Geometry: final body of the model. Coordinates: model frame, mm. A direction names the side the tool comes from. Coordinates: 2 decimals unless noted, no trailing zeros. Order: outer loops, then holes, each group sorted by start corner. A loop starts at its lowest first (then second) coordinate and runs counter-clockwise, first axis right, second up. Notation, with made-up numbers: (61, 85.5) - (80, 85.5) arc R32 ccw to (80, 113.5) - close; hole circle Ø9 at (-2.5, 69.5). An arc over 180 degrees is marked (long way). Use a Markdown table: item, result. Add a question column.
```python
from build123d import *

# Parameters (mm, degrees)
CROQUIS1_W              = 50
CROQUIS1_H              = 50
CROQUIS1_W_2            = 40
CROQUIS1_H_2            = 40
SALIENTE_EXTRUIR1_DEPTH = 25
CROQUIS2_R              = 8
CORTAR_EXTRUIR1_DEPTH   = 60
CROQUIS3_R              = 8
CORTAR_EXTRUIR2_DEPTH   = 60


with BuildPart() as part:
    # Croquis1 → Saliente-Extruir1 (new body)
    with BuildSketch(Plane.XY):
        Rectangle(CROQUIS1_W, CROQUIS1_H)
        Rectangle(CROQUIS1_W_2, CROQUIS1_H_2, mode=Mode.SUBTRACT)
    extrude(amount=SALIENTE_EXTRUIR1_DEPTH)

    # Croquis2 → Cortar-Extruir1 (cut)
    with BuildSketch(Plane(origin=(0, 25, 0), x_dir=(1, 0, 0), z_dir=(0, 1, 0))):
        with Locations(Location((0, -12.5, 0), (0, 0, 270))):
            Circle(CROQUIS2_R)
    extrude(amount=-CORTAR_EXTRUIR1_DEPTH, mode=Mode.SUBTRACT)

    # Croquis3 → Cortar-Extruir2 (cut)
    with BuildSketch(Plane(origin=(25, 0, 0), x_dir=(0, 0, -1), z_dir=(1, 0, 0))):
        with Locations(Location((-12.5, 0, 0), (0, 0, 90))):
            Circle(CROQUIS3_R)
    extrude(amount=-CORTAR_EXTRUIR2_DEPTH, mode=Mode.SUBTRACT)


solid = part.part
```
1) Section query A-A (x = 0). Return the cut outline in (y, z).
2) Line query: line 1 (Y direction, x = -9, z = 15.5); line 2 (X direction, y = -22.55, z = 12.5). Output: solid intervals per line, ascending. Write a range as from..to.
3) Access query for faces 4 (the cylindrical face through (-22.47, -1.73, 4.69)), 5 (the flat face through (0, -20, 21)). Directions: +Z, -Z, +X, -X, +Y, -Y. A direction counts if a zero-diameter tool reaches every point of the face in a straight line with its end or side. Return the directions, or none.
4) Section query B-B (y = 12). Return the cut outline in (x, z).
5) Draft query along Z for faces 1 (the flat face through (-23, 0, 0)), 2 (the flat face through (-5.9, 25, 6.8)), 3 (the cylindrical face through (-7.81, 22.54, 10.77)). Return one class per face: released by +Z, released by -Z, zero draft, split by the parting line, or undercut.
6) Section query D-D (z = 12.5). Return the cut outline in (x, y).
From the geometry:
| question | item | result |
|---|---|---|
| 1 | outline | (-25, 0) - (-20, 0) - (-20, 4.5) - (-25, 4.5) - close; (-25, 20.5) - (-20, 20.5) - (-20, 25) - (-25, 25) - close; (20, 0) - (25, 0) - (25, 4.5) - (20, 4.5) - close; (20, 20.5) - (25, 20.5) - (25, 25) - (20, 25) - close |
| 2 | line 1 | y = -25..-20, 20..25 |
| 2 | line 2 | x = -25..-8, 8..25 |
| 3 | face 4 | +X, -X |
| 3 | face 5 | +Z, -Z |
| 4 | outline | (-25, 0) - (-20, 0) - (-20, 25) - (-25, 25) - close; (20, 0) - (25, 0) - (25, 25) - (20, 25) - close |
| 5 | face 1 | released by -Z |
| 5 | face 2 | zero draft |
| 5 | face 3 | undercut |
| 6 | outline | (-25, -25) - (-8, -25) - (-8, -20) - (-20, -20) - (-20, -8) - (-25, -8) - close; (-25, 8) - (-20, 8) - (-20, 20) - (-8, 20) - (-8, 25) - (-25, 25) - close; (8, -25) - (25, -25) - (25, -8) - (20, -8) - (20, -20) - (8, -20) - close; (8, 20) - (20, 20) - (20, 8) - (25, 8) - (25, 25) - (8, 25) - close |
